Could you check a few things on this model? Use its own coordinates, in mm. A direction names the side the tool comes from. Give positions to 0.01 mm unless a question says otherwise; leave off trailing zeros. Write each loop counter-clockwise with the first axis right and the second up, starting at its lowest first coordinate (ties: lowest second). Pieces come first, ordered by that corner, then holes. Notation, with made-up numbers: M 83,28.5 L 123,28.5 A25 cw 123,51.5 Z; hole C 36,78.5 d11. An arc over 180 degrees is marked long. Answer as CSV lines item,"result". Start each with the question number.
from build123d import *

# Parameters (mm, degrees)
SKETCH_W      = 60
SKETCH_H      = 40
SKETCH_R      = 1
PAD_DEPTH     = 2
SKETCH001_W   = 10.734469
SKETCH001_H   = 6
SKETCH001_W_2 = 6
SKETCH001_H_2 = 18.785311
SKETCH001_W_3 = 40.960449
SKETCH001_W_4 = 9.745754
PAD001_DEPTH  = 5


with BuildPart() as part:
    # Sketch → Pad (new body)
    with BuildSketch(Plane.YZ):
        with Locations((30, 20)):
            Rectangle(SKETCH_W, SKETCH_H)
        with Locations((3.035, 34.678047)):
            Circle(SKETCH_R, mode=Mode.SUBTRACT)
        with Locations((56.965, 34.678047)):
            Circle(SKETCH_R, mode=Mode.SUBTRACT)
        with Locations((56.965, 4.678047)):
            Circle(SKETCH_R, mode=Mode.SUBTRACT)
        with Locations((3.035, 4.678047)):
            Circle(SKETCH_R, mode=Mode.SUBTRACT)
    extrude(amount=PAD_DEPTH)

    # Sketch001 (on Face10 of Pad) → Pad001 (join)
    with BuildSketch(Plane.YZ.offset(2)):
        with Locations((13.569118, 34.265322)):
            Rectangle(SKETCH001_W, SKETCH001_H)
        with Locations((55.642065, 20.339975)):
            Rectangle(SKETCH001_W_2, SKETCH001_H_2)
        with Locations((28.823356, 5.767194)):
            Rectangle(SKETCH001_W_3, SKETCH001_H)
        with Locations((42.696971, 34.192021)):
            Rectangle(SKETCH001_W_4, SKETCH001_H)
    extrude(amount=PAD001_DEPTH)


solid = part.part
1. Imagine slicing it at B-B, the plane y = 12. Please give me the cut outline in (x, z), plus the area to 3 significant figures.
2. Imagine slicing it at C-C, the plane z = 22. Please give me the cut outline in (x, y).
3. Please list where these lines run through material, in increasing order: line 1 (Z direction, x = 5, y = 10.5); line 2 (Z direction, x = 3, y = 46); line 3 (X direction, y = 44.5, z = 26.5).
4. Imagine slicing it at D-D, the plane y = 26. Please give me the cut outline in (x, z).
5. Imagine slicing it at A-A, the plane x = 4. Please give me the cut outline in (y, z).
6. Thinking about a two-plate mould opening in Y: for faces 5 (the flat face through (4, 43, 31.192)), 6 (the flat face through (4, 18.936, 34)), 7 (the flat face through (1, 60, 20)), 8 (the flat face through (4, 52.642, 20)), which applies, pulls with the +Y half, pulls with the -Y half, needs draft (parallel to the pull), parting line crosses it, or undercut?
7. Will these pins go through, and if not, where does the flat tip stop? P1, Ø1.5, axis at x = 3.5, z = 34, coming from the +Y side; P2, Ø1.5, axis at x = 4, y = 16, coming from the -Z side; P3, Ø1.5, axis at x = 3.5, z = 22.5, coming from the -Y side.
8. On a 3-axis mill with a long thin cutter (end or side, diameter ignored), from which of +Z, -Z, +X, -X, +Y, -Y can I reach the whole of each face in a straight line? I mean faces 1 (the flat face through (4, 37.824, 34)), 2 (the flat face through (4, 13, 31.265)), 3 (the flat face through (4, 29, 8.767)), 4 (the flat face through (4, 43, 37.192)). Say none if no direction works.
Solutions:
1,outline,"M 0,0 L 2,0 L 2,2.77 L 7,2.77 L 7,8.77 L 2,8.77 L 2,31.27 L 7,31.27 L 7,37.27 L 2,37.27 L 2,40 L 0,40 Z"
1,area,"140 mm²"
2,outline,"M 0,0 L 2,0 L 2,52.64 L 7,52.64 L 7,58.64 L 2,58.64 L 2,60 L 0,60 Z"
3,line 1,"2.77 to 8.77, 31.27 to 37.27"
3,line 2,"2.77 to 8.77, 31.19 to 37.19"
3,line 3,"0 to 2"
4,outline,"M 0,0 L 2,0 L 2,2.77 L 7,2.77 L 7,8.77 L 2,8.77 L 2,40 L 0,40 Z"
5,outline,"M 8.2,31.27 L 18.94,31.27 L 18.94,37.27 L 8.2,37.27 Z; M 8.34,2.77 L 49.3,2.77 L 49.3,8.77 L 8.34,8.77 Z; M 37.82,31.19 L 47.57,31.19 L 47.57,37.19 L 37.82,37.19 Z; M 52.64,10.95 L 58.64,10.95 L 58.64,29.73 L 52.64,29.73 Z"
6,face 5,"needs draft"
6,face 6,"undercut"
6,face 7,"pulls with the +Y half"
6,face 8,"pulls with the -Y half"
7,P1,"y = 47.57"
7,P2,"z = 2.77"
7,P3,"y = 52.64"
8,face 1,"+Z, +X"
8,face 2,"+X, -Y"
8,face 3,"+X, +Y, -Y"
8,face 4,"+Z, +X, +Y"
